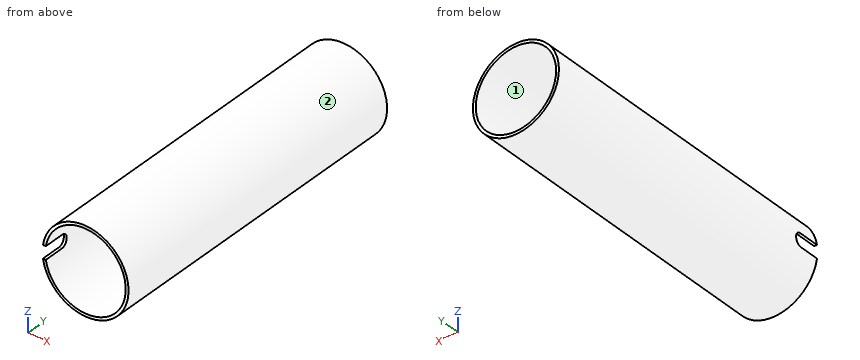
Autodesk Inventor part; units mm, degrees
ref_plane "YZ Plane" through (0, 0, 0) normal (1, 0, 0) x (0, 1, 0)
ref_plane "XZ Plane" through (0, 0, 0) normal (0, 1, 0) x (-1, 0, 0)
ref_plane "XY Plane" through (0, 0, 0) normal (0, 0, 1) x (1, 0, 0)
sketch "Sketch1" plane through (0, 0, 0) normal (0, 1, 0) x (-1, 0, 0)
  circle A0 centre (0, 0) radius 50
  circle A1 centre (0, 0) radius 53.5
  dimension "d0" = 100
  dimension "d1" = 3.5
extrude "Extrusion1" add sketch "Sketch1" along normal blind 400
sketch "Sketch3" plane through (0, 0, 0) normal (1, 0, 0) x (0, 1, 0)
  spline S0 degree 3 poles (25, -8) (26.0064, -8) (27.0786, -7.7985) (29.0491, -6.9816) (29.9475, -6.3662) (31.3662, -4.9476) (31.9816, -4.0491) (32.7985, -2.0786) (33, -1.0063) (33, 1.0063) (32.7985, 2.0786) (31.9816, 4.0491) (31.3662, 4.9476) (29.9475, 6.3662) (29.0491, 6.9816) (27.0786, 7.7985) (26.0064, 8) (25, 8) knots -2.41526 -2.41526 -2.41526 -2.41526 -2.113349 -2.113349 -1.811438 -1.811438 -1.509534 -1.509534 -1.20763 -1.20763 -0.905726 -0.905726 -0.603822 -0.603822 -0.301911 -0.301911 0 0 0 0
  line L0 (25, 8) -> (0, 8)
  line L1 (0, -8) -> (25, -8)
  line L2 (0, 8) -> (0, -8)
  line L3 (0, 53.5) -> (0, -53.5)
  point P0 (0, 0)
extrude "Extrusion2" cut sketch "Sketch3" against normal through all
properties part number "Crusher_Tube"
Work out the finished part from the listing and answer in its coordinate system (mm). Face numbers are marked on the shaded views. Round coordinates to 2 decimals unless told otherwise and drop trailing zeros. Write each loop counter-clockwise with the first axis right and the second up, starting at its lowest first coordinate (ties: lowest second). Pieces come first, ordered by that corner, then holes. Notation, with made-up numbers: (62, 41) - (113, 41) arc R25 ccw to (113, 68) - close; hole circle Ø10 at (15.5, -4). An arc over 180 degrees is marked (long way). Return JSON: item names as keys, results as strings. Group by question number.
Q1. The part is cut by section B-B on x = 0. Write down the section's boundary in (y, z).
Q2. The part is cut by section A-A on z = 38.5. Write down the section's boundary in (x, y), then the cut area to 3 significant figures.
Q3. The part is cut by section C-C on y = 138.5. Write down the section's boundary in (x, z), then the cut area to 3 significant figures.
Q4. Find the intervals of material crossed by L1, parallel to Z at x = 0, y = 208; L2, parallel to X at y = 280, z = -44, in increasing order.
Q5. Each of these flat-tipped pins is pushed along its axis until it touches: pin 1 Ø12 at (y, z) = (266, -24) entering from +X; pin 2 Ø1 at (x, y) = (2, 177.5) entering from +Z; pin 3 Ø6 at (y, z) = (320, 30) entering from +X. Where does it stop, or does it pass through?
Q6. The mould has two halves that part along Z. Classify the marked faces 1 and 2: released by +Z, released by -Z, zero draft, split by the parting line, or undercut.
Solved:
{
 "1": {"outline": "(0, -53.5) - (400, -53.5) - (400, -50) - (0, -50) - close; (0, 50) - (400, 50) - (400, 53.5) - (0, 53.5) - close"},
 "2": {"outline": "(-37.15, 0) - (-31.9, 0) - (-31.9, 400) - (-37.15, 400) - close; (31.9, 0) - (37.15, 0) - (37.15, 400) - (31.9, 400) - close", "area": "4,200 mm²"},
 "3": {"outline": "circle Ø107 at (0, 0); hole circle Ø100 at (0, 0)", "area": "1,140 mm²"},
 "4": {"L1": "-53.5 to -50, 50 to 53.5", "L2": "-30.43 to -23.75, 23.75 to 30.43"},
 "5": {"pin 1": "x = 50.38", "pin 2": "z = 53.48", "pin 3": "x = 46.19"},
 "6": {"face 1": "undercut", "face 2": "split by the parting line"}
}
